from build123d import *

# Parameters (mm, degrees)
CROQUIS1_W            = 8.9
CROQUIS1_H            = 25
CROQUIS2_R            = 6
CORTAR_EXTRUIR1_DEPTH = 17
CROQUIS3_R            = 3
CORTAR_EXTRUIR2_DEPTH = 12.5


with BuildPart() as part:
    # Croquis1 → Revolución1 (revolve)
    with BuildSketch(Plane.XY):
        with Locations((4.45, 12.5)):
            Rectangle(CROQUIS1_W, CROQUIS1_H)
    revolve(axis=Axis((0, 0, 0), (0, 1, 0)))

    # Croquis2 → Cortar-Extruir1 (cut)
    with BuildSketch(Plane(origin=(0, 25, 0), x_dir=(1, 0, 0), z_dir=(0, 1, 0))):
        with Locations(Location((0, 0, 0), (0, 0, 180))):
            Circle(CROQUIS2_R)
    extrude(amount=-CORTAR_EXTRUIR1_DEPTH, mode=Mode.SUBTRACT)

    # Croquis3 → Cortar-Extruir2 (cut)
    with BuildSketch(Plane.XZ):
        Circle(CROQUIS3_R)
    extrude(amount=-CORTAR_EXTRUIR2_DEPTH, mode=Mode.SUBTRACT)


solid = part.part
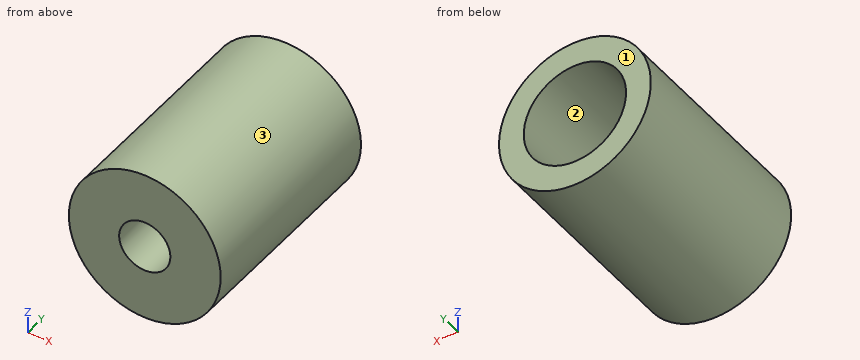
CAD build for the part. Positions are in the model's coordinates, mm. Face numbers are marked on the shaded views. Round coordinates to 2 decimals unless told otherwise and drop trailing zeros. Loops run counter-clockwise (first coordinate to the right, second up) from the corner with the lowest first, then second, coordinate; pieces in that order, holes last.
(1) Cut at A-A (z = 0). Give the cut face in (x, y), plus the area to 3 significant figures.
(2) Cut at D-D (x = -4). Give the cut face in (y, z).
(3) Cut at B-B (x = 0). Give the cut face in (y, z), plus the area to 3 significant figures.
(4) Drop flat-ended pins along their axis: pin 1 (2 mm diameter, centred on y = 8, z = -6, fed in from +X); pin 2 (1.5 mm diameter, centred on y = 16.5, z = 1.5, fed in from +X); pin 3 (9.5 mm diameter, centred on x = 0, z = 0, fed in from +Y). Give the stop position or say it passes through.
(5) Two-plate mould, pull along X, no slides. Class the marked faces 1, 2 and 3: +X half, -X half, draft (parallel to the pull), parting line (faces both ways), or undercut.
(6) Wall check: line 1 along Z through (x, y) = (0, 3.5); line 2 along Z through (x, y) = (0, 14.75); line 3 along Y through (x, z) = (5.5, 1). Give the ranges that are in metal, low to high.
(7) Cut at C-C (y = 13.25). Give the cut face in (x, z).
Findings below:
1. outline: (-8.9, 0) - (-3, 0) - (-3, 8) - (-6, 8) - (-6, 25) - (-8.9, 25) - close; (3, 0) - (8.9, 0) - (8.9, 25) - (6, 25) - (6, 8) - (3, 8) - close
1. area: 193 mm2
2. outline: (0, -7.95) - (25, -7.95) - (25, -4.47) - (8, -4.47) - (8, 4.47) - (25, 4.47) - (25, 7.95) - (0, 7.95) - close
3. outline: (0, -8.9) - (25, -8.9) - (25, -6) - (8, -6) - (8, -3) - (0, -3) - close; (0, 3) - (8, 3) - (8, 6) - (25, 6) - (25, 8.9) - (0, 8.9) - close
3. area: 193 mm2
4. pin 1: stops at x = 7.36
4. pin 2: stops at x = 8.87
4. pin 3: stops at y = 8
5. face 1: draft
5. face 2: undercut
5. face 3: parting line
6. line 1: z = -8.9 to -3, 3 to 8.9
6. line 2: z = -8.9 to -6, 6 to 8.9
6. line 3: y = 0 to 8
7. outline: circle Ø17.8 at (0, 0); hole circle Ø12 at (0, 0)
